```python
from build123d import *

# Parameters (mm, degrees)
SKETCH2_R           = 4
BOSS_EXTRUDE1_DEPTH = 7
SKETCH3_R           = 5
BOSS_EXTRUDE2_DEPTH = 5
SKETCH4_R           = 1.65
CUT_EXTRUDE1_DEPTH  = 12
SKETCH5_R           = 2
CUT_EXTRUDE2_DEPTH  = 5


with BuildPart() as part:
    # Sketch2 → Boss-Extrude1 (new body)
    with BuildSketch(Plane(origin=(0, 0, 0), x_dir=(1, 0, 0), z_dir=(0, 1, 0))):
        Circle(SKETCH2_R)
    extrude(amount=BOSS_EXTRUDE1_DEPTH)

    # Sketch3 → Boss-Extrude2 (add)
    with BuildSketch(Plane.XZ):
        Circle(SKETCH3_R)
    extrude(amount=BOSS_EXTRUDE2_DEPTH)

    # Sketch4 → Cut-Extrude1 (cut)
    with BuildSketch(Plane(origin=(0, 7, 0), x_dir=(1, 0, 0), z_dir=(0, 1, 0))):
        Circle(SKETCH4_R)
    extrude(amount=-CUT_EXTRUDE1_DEPTH, mode=Mode.SUBTRACT)

    # Sketch5 → Cut-Extrude2 (cut)
    with BuildSketch(Plane.XZ.offset(-7)):
        Circle(SKETCH5_R)
    extrude(amount=CUT_EXTRUDE2_DEPTH, mode=Mode.SUBTRACT)


solid = part.part
```
Geometry check sheet. Reference: the model listing, model coordinates, mm. A direction names the side the tool comes from. Round coordinates to 2 decimals unless told otherwise and drop trailing zeros. Order: outer loops, then holes, each group sorted by start corner. A loop starts at its lowest first (then second) coordinate and runs counter-clockwise, first axis right, second up. Notation, with made-up numbers: (66, 67) - (77, 67) arc R14 ccw to (77, 72) - close; hole circle Ø9 at (-18.75, 47). An arc over 180 degrees is marked (long way). Use a Markdown table: item, result. Add a question column.
1) Section check C-C (y = 6). Record the cut outline in (x, z), then the cut area to 3 significant figures.
2) Mould release check, pull along X, two halves, no side actions. Record for faces 3 (the cylindrical face through (-1.08, -2.46, -4.88)), 4 (the flat face through (2, -5, 0)), 5 (the cylindrical face through (-1.216, -1.451, -1.115)): released by +X, released by -X, zero draft, split by the parting line, or undercut.
3) Section check A-A (z = 0). Record the cut outline in (x, y).
4) Set-up check for faces 1 (the flat face through (-2, 7, 1)), 2 (the cylindrical face through (-0.867, 3.451, 3.905)): record each of +Z, -Z, +X, -X, +Y, -Y from which the full face is reachable in a straight line by a thin tool's end or side.
5) Section check B-B (x = 0). Record the cut outline in (y, z), then the cut area to 3 significant figures.
6) Thickness scan on line 1 along X through (y, z) = (1.5, 0); line 2 along Z through (x, y) = (0, 3.4); line 3 along Z through (x, y) = (0, -0.5). Record the ranges inside material, lowest first.
7) Section check D-D (z = 3.5). Record the cut outline in (x, y).
8) Gauge pin test, flat ends, axial feed: P1, Ø1, axis at y = 5, z = -3.5, coming from the +X side; P2, Ø1.5, axis at x = -1, y = -3.5, coming from the +Z side. Record the tip position at first contact, or that the pin passes through.
Established:
| question | item | result |
|---|---|---|
| 1 | outline | circle Ø8 at (0, 0); hole circle Ø4 at (0, 0) |
| 1 | area | 37.7 mm2 |
| 2 | face 3 | split by the parting line |
| 2 | face 4 | zero draft |
| 2 | face 5 | undercut |
| 3 | outline | (-5, -5) - (-1.65, -5) - (-1.65, 2) - (-2, 2) - (-2, 7) - (-4, 7) - (-4, 0) - (-5, 0) - close; (1.65, -5) - (5, -5) - (5, 0) - (4, 0) - (4, 7) - (2, 7) - (2, 2) - (1.65, 2) - close |
| 4 | face 1 | +Z, -Z, +X, -X, +Y |
| 4 | face 2 | +Y |
| 5 | outline | (-5, -5) - (0, -5) - (0, -4) - (7, -4) - (7, -2) - (2, -2) - (2, -1.65) - (-5, -1.65) - close; (-5, 1.65) - (2, 1.65) - (2, 2) - (7, 2) - (7, 4) - (0, 4) - (0, 5) - (-5, 5) - close |
| 5 | area | 62.9 mm2 |
| 6 | line 1 | -4 to -1.65, 1.65 to 4 |
| 6 | line 2 | -4 to -2, 2 to 4 |
| 6 | line 3 | -5 to -1.65, 1.65 to 5 |
| 7 | outline | (-3.57, -5) - (3.57, -5) - (3.57, 0) - (1.94, 0) - (1.94, 7) - (-1.94, 7) - (-1.94, 0) - (-3.57, 0) - close |
| 8 | P1 | x = 2.65 |
| 8 | P2 | z = 4.99 |
